Source: CAD feature listing. Evaluate the final solid. Frame: model axes, mm. Face numbers are marked on the shaded views. Round coordinates to 2 decimals unless told otherwise and drop trailing zeros. Order: outer loops, then holes, each group sorted by start corner. A loop starts at its lowest first (then second) coordinate and runs counter-clockwise, first axis right, second up. Notation, with made-up numbers: (-13.5, -22) -> (42.5, -22) arc R34 cw to (42.5, 14) -> close; hole circle Ø1 at (45, 42.25). An arc over 180 degrees is marked (long way). Answer as CSV lines item,"result". Start each with the question number.
(1) Section query C-C (y = -51.5). Output: boundary loops of the cut face in (x, z), plus the area to 3 significant figures.
(2) Contact query for a flat-ended pin moving along its axis: P1, Ø1.2, axis at x = -84.5, z = 3, coming from the +Y side. Output: stop coordinate, or through.
(3) Pull-direction query (Z, two-part tool) for the marked faces 1 and 2; classes: +Z half, -Z half, draft (parallel to the pull), parting line (faces both ways), or undercut.
(4) Section query B-B (x = 0). Output: boundary loops of the cut face in (y, z).
(5) Section query D-D (x = -78.5). Output: boundary loops of the cut face in (y, z).
(6) Line query: line 1 along Y through (x, z) = (-218, 2.6); line 2 along X through (y, z) = (-65, 1); line 3 along X through (y, z) = (0.5, 1.5). Output: solid intervals per line, ascending. Write a range as from..to.
(7) Section query A-A (z = 3.3). Count the separate pieces of the cut face and the enclosed holes in it, plus the area to 3 significant figures.
```python
from build123d import *

# Parameters (mm, degrees)
ESQUISSE1_W             = 440
ESQUISSE1_H             = 150
BOSS_EXTRU_1_DEPTH      = 4
ESQUISSE2_R             = 11
ENL_V_MAT_EXTRU_1_DEPTH = 10
ESQUISSE3_W             = 3.624864112
ESQUISSE3_H             = 60
ESQUISSE3_W_2           = 4.375135888
ESQUISSE3_W_3           = 50
ESQUISSE3_H_2           = 4
ENL_V_MAT_EXTRU_2_DEPTH = 4
ESQUISSE4_R             = 1.6
ENL_V_MAT_EXTRU_3_DEPTH = 4


with BuildPart() as part:
    # Esquisse1 → Boss.-Extru.1 (new body)
    with BuildSketch(Plane.XY):
        Rectangle(ESQUISSE1_W, ESQUISSE1_H)
    extrude(amount=BOSS_EXTRU_1_DEPTH)

    # Esquisse2 → Enlèv. mat.-Extru.1 (cut)
    with BuildSketch(Plane(origin=(0, 0, 0), x_dir=(-1, 0, 0), z_dir=(0, 0, -1))):
        Circle(ESQUISSE2_R)
    extrude(amount=-ENL_V_MAT_EXTRU_1_DEPTH, mode=Mode.SUBTRACT)

    # Esquisse3 → Enlèv. mat.-Extru.2 (cut)
    with BuildSketch(Plane(origin=(0, 0, 0), x_dir=(-1, 0, 0), z_dir=(0, 0, -1))):
        with Locations((218.187567944, -30)):
            Rectangle(ESQUISSE3_W, ESQUISSE3_H)
        with Locations((-217.812432056, -30)):
            Rectangle(ESQUISSE3_W_2, ESQUISSE3_H)
        with Locations((95.375135888, 73)):
            Rectangle(ESQUISSE3_W_3, ESQUISSE3_H_2)
        with Locations((-94.624864112, 73)):
            Rectangle(ESQUISSE3_W_3, ESQUISSE3_H_2)
    extrude(amount=-ENL_V_MAT_EXTRU_2_DEPTH, mode=Mode.SUBTRACT)

    # Esquisse4 → Enlèv. mat.-Extru.3 (cut)
    with BuildSketch(Plane(origin=(0, 0, 0), x_dir=(-1, 0, 0), z_dir=(0, 0, -1))):
        with Locations((-217.624864112, 14)):
            Circle(ESQUISSE4_R)
        with Locations((-218, 73)):
            Circle(ESQUISSE4_R)
        with Locations((-218, -65)):
            Circle(ESQUISSE4_R)
        with Locations((-133.624864112, 73)):
            Circle(ESQUISSE4_R)
        with Locations((-55.624864112, 73)):
            Circle(ESQUISSE4_R)
        with Locations(Location((55.624864112, 73, 0), (0, 0, 180))):
            Circle(ESQUISSE4_R)
        with Locations(Location((133.624864112, 73, 0), (0, 0, 180))):
            Circle(ESQUISSE4_R)
        with Locations(Location((218, -65, 0), (0, 0, 180))):
            Circle(ESQUISSE4_R)
        with Locations(Location((218, 73, 0), (0, 0, 180))):
            Circle(ESQUISSE4_R)
        with Locations(Location((217.624864112, 14, 0), (0, 0, 180))):
            Circle(ESQUISSE4_R)
    extrude(amount=-ENL_V_MAT_EXTRU_3_DEPTH, mode=Mode.SUBTRACT)


solid = part.part
```
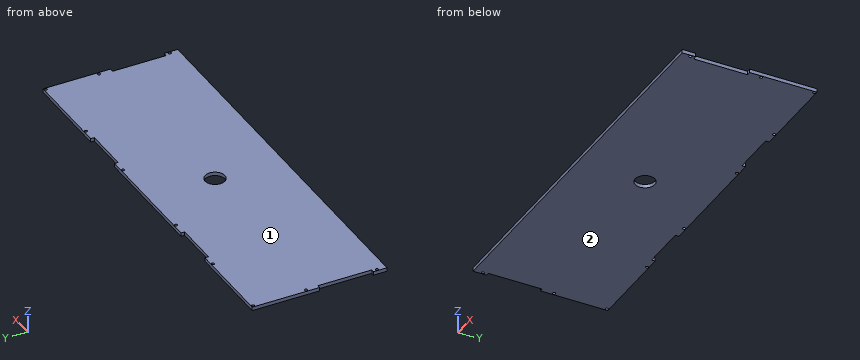
Answer block:
1,outline,"(-216.38, 0) -> (215.62, 0) -> (215.62, 4) -> (-216.38, 4) -> close"
1,area,"1,730 mm2"
2,P1,"y = 71"
3,face 1,"+Z half"
3,face 2,"-Z half"
4,outline,"(-75, 0) -> (-11, 0) -> (-11, 4) -> (-75, 4) -> close; (11, 0) -> (75, 0) -> (75, 4) -> (11, 4) -> close"
5,outline,"(-75, 0) -> (71, 0) -> (71, 4) -> (-75, 4) -> close"
6,line 1,"-75..-66.6, -63.4..-60, 0..12.44, 15.56..71.4, 74.6..75"
6,line 2,"-220..-219.6, -216.4..216.4, 219.6..220"
6,line 3,"-220..-10.99, 10.99..220"
7,separate pieces,"1"
7,enclosed holes,"11"
7,area,"64,700 mm2"
